Check sheet for the modelled part. Datum: model origin and axes. Units: mm. Give positions to 0.01 mm unless a question says otherwise; leave off trailing zeros. Write each question's results on one line, items separated by ' | '. Start each with the question number.
```python
from build123d import *

# Parameters (mm, degrees)
SKETCH1_W                        = 127
SKETCH1_H                        = 50.8
BOSS_EXTRUDE1_DEPTH              = 3.175
F_17_64_0_26563_DIAMETER_HOLE1_D = 6.747002
F_17_64_0_26563_DIAMETER_HOLE2_D = 6.747002


with BuildPart() as part:
    # Sketch1 → Boss-Extrude1 (new body)
    with BuildSketch(Plane.XY):
        with Locations((-11.921727019, 3.749860724)):
            Rectangle(SKETCH1_W, SKETCH1_H)
    extrude(amount=BOSS_EXTRUDE1_DEPTH)

    # 17/64 (0.26563) Diameter Hole1 (through all)
    with Locations(Plane(origin=(-43.671727019, 19.624860724, 3.175), x_dir=(1, 0, 0), z_dir=(0, 0, 1))):
        with Locations((0, 0), (0, -31.75), (89.2175, 0), (89.2175, -31.75)):
            Hole(F_17_64_0_26563_DIAMETER_HOLE1_D / 2)

    # 17/64 (0.26563) Diameter Hole2 (through all)
    with Locations(Plane(origin=(-69.071727019, 22.799860724, 3.175), x_dir=(1, 0, 0), z_dir=(0, 0, 1))):
        with Locations((0, 0), (12.7, 0), (12.7, -38.1), (0, -38.1)):
            Hole(F_17_64_0_26563_DIAMETER_HOLE2_D / 2)


solid = part.part
```
Item 1: Depth check by flat-ended pin: pin 1 Ø6 at (x, y) = (-43.67, 19.62) entering from -Z. Enter the tip coordinate at first touch or a pass-through.
Item 2: Mould release check, pull along Y, two halves, no side actions. Record for faces 1 (the flat face through (51.578, 3, 2)), 2 (the cylindrical face through (-65.7, -15.2, 1.6)), 3 (the flat face through (-13, 29.15, 2)), 4 (the flat face through (-13, -21.65, 2)): pulls with the +Y half, pulls with the -Y half, needs draft (parallel to the pull), parting line crosses it, or undercut.
Item 3: Thickness scan on probe 1 along X at (y, z) = (-18, 1.55); probe 2 along X at (y, z) = (21, 0.45); probe 3 along X at (y, z) = (17, 3). Record the ranges inside material, lowest first. Write a range as from..to.
Item 4: Section check A-A on z = 1.7. Count the separate pieces of the cut face and the enclosed holes in it, then the cut area to 3 significant figures.
Check sheet entries:
1) pin 1: passes through
2) face 1: needs draft | face 2: undercut | face 3: pulls with the +Y half | face 4: pulls with the -Y half
3) probe 1: x = -75.42..-71.09, -67.05..-58.39, -54.35..51.58 | probe 2: x = -75.42..-71.92, -66.22..-59.22, -53.52..-46.75, -40.59..42.47, 48.63..51.58 | probe 3: x = -75.42..-45.79, -41.55..43.43, 47.66..51.58
4) separate pieces: 1 | enclosed holes: 8 | area: 6,170 mm^2
